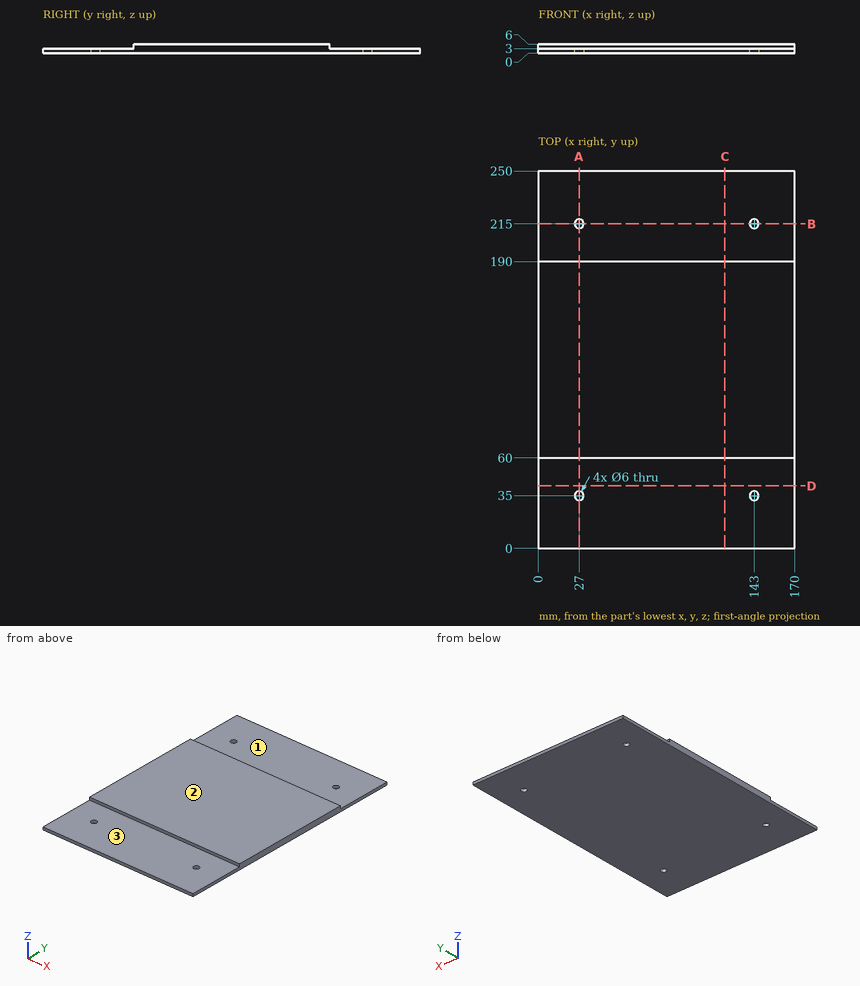
Verification items for this drawing (mm, ordinates from the low corner). A direction names the side the tool comes from. Coordinates: 2 decimals unless noted, no trailing zeros. Loops run counter-clockwise (first coordinate to the right, second up) from the corner with the lowest first, then second, coordinate; pieces in that order, holes last. Notation, with made-up numbers: (-18.5, 33) -> (13.5, 33) arc R30 cw to (13.5, 69) -> close; hole circle Ø7 at (-24, -30.75). An arc over 180 degrees is marked (long way). Put each result on its own line as item: value.
1. Gauge pin test, flat ends, axial feed: P1, Ø7, axis at x = 143, y = 35, coming from the -Z side; P2, Ø3.5, axis at x = 85.5, z = 5, coming from the +Y side; P3, Ø6, axis at x = 122.5, y = 38.5, coming from the +Z side; P4, Ø0.9, axis at x = 61.5, z = 4.5, coming from the -Y side. Record the tip position at first contact, or that the pin passes through.
Result set:
P1: stops at z = 0
P2: stops at y = 190
P3: stops at z = 3
P4: stops at y = 60
2. Thickness scan on line 1 (Y direction, x = 27, z = 2); line 2 (X direction, y = 215, z = 1.3); line 3 (Z direction, x = 148, y = 46). Record the ranges inside material, lowest first.
Result set:
line 1: y = 0 to 32, 38 to 212, 218 to 250
line 2: x = 0 to 24, 30 to 140, 146 to 170
line 3: z = 0 to 3
3. Section check B-B, the plane y = 215. Record the boundary of the cut face in (x, z).
Result set:
outline: (0, 0) -> (24, 0) -> (24, 3) -> (0, 3) -> close; (30, 0) -> (140, 0) -> (140, 3) -> (30, 3) -> close; (146, 0) -> (170, 0) -> (170, 3) -> (146, 3) -> close
4. Tool access check on the marked faces 1, 2 and 3. Record the directions out of +Z, -Z, +X, -X, +Y, -Y that give a thin tool (end or side, any length) a straight path to the whole face; none if there is none.
Result set:
face 1: +Z, +X, -X, +Y
face 2: +Z, +X, -X, +Y, -Y
face 3: +Z, +X, -X, -Y
5. Section check D-D, the plane y = 41.5. Record the boundary of the cut face in (x, z), then the cut area to 3 significant figures.
Result set:
outline: (0, 0) -> (170, 0) -> (170, 3) -> (0, 3) -> close
area: 510 mm^2
6. Section check C-C, the plane x = 123.5. Record the boundary of the cut face in (y, z), then the cut area to 3 significant figures.
Result set:
outline: (0, 0) -> (250, 0) -> (250, 3) -> (190, 3) -> (190, 6) -> (60, 6) -> (60, 3) -> (0, 3) -> close
area: 1,140 mm^2
7. Section check A-A, the plane x = 27. Record the boundary of the cut face in (y, z), then the cut area to 3 significant figures.
Result set:
outline: (0, 0) -> (32, 0) -> (32, 3) -> (0, 3) -> close; (38, 0) -> (212, 0) -> (212, 3) -> (190, 3) -> (190, 6) -> (60, 6) -> (60, 3) -> (38, 3) -> close; (218, 0) -> (250, 0) -> (250, 3) -> (218, 3) -> close
area: 1,100 mm^2
